Here's how the part is built. I have some questions about the finished solid (model axes, mm). A direction names the side the tool comes from. Coordinates: 2 decimals unless noted, no trailing zeros. Write each loop counter-clockwise with the first axis right and the second up, starting at its lowest first coordinate (ties: lowest second). Pieces come first, ordered by that corner, then holes. Notation, with made-up numbers: (-36, 39.25) -> (-19, 39.25) arc R21 cw to (-19, 76.25) -> close; hole circle Ø4 at (35.25, -34). An arc over 180 degrees is marked (long way). Use a Markdown table: item, result. Add a question column.
```python
from build123d import *

# Parameters (mm, degrees)
SKETCH1_W           = 7
SKETCH1_H           = 6
BOSS_EXTRUDE1_DEPTH = 9
SKETCH2_W           = 2
SKETCH2_H           = 2
SKETCH2_W_2         = 1
SKETCH2_H_2         = 3
CUT_EXTRUDE1_DEPTH  = 7
SKETCH3_OUTSIDE_W   = 11.576
SKETCH3_OUTSIDE_H   = 13.576
CUT_EXTRUDE3_DEPTH  = 3
CUT_EXTRUDE4_DEPTH  = 3
CUT_EXTRUDE5_DEPTH  = 1
SKETCH8_W           = 3
SKETCH8_H           = 3.605551275
CUT_EXTRUDE6_DEPTH  = 5.160251472


with BuildPart() as part:
    # Sketch1 → Boss-Extrude1 (new body)
    with BuildSketch(Plane.XY):
        Rectangle(SKETCH1_W, SKETCH1_H)
    extrude(amount=BOSS_EXTRUDE1_DEPTH)

    # Sketch2 → Cut-Extrude1 (cut, through all)
    with BuildSketch(Plane(origin=(0, 3, 0), x_dir=(1, 0, 0), z_dir=(0, 1, 0))):
        with Locations((-2.5, -8)):
            Rectangle(SKETCH2_W, SKETCH2_H)
        with Locations((2.5, -8)):
            Rectangle(SKETCH2_W, SKETCH2_H)
        with Locations((3, -3.5)):
            Rectangle(SKETCH2_W_2, SKETCH2_H_2)
    extrude(amount=-CUT_EXTRUDE1_DEPTH, mode=Mode.SUBTRACT)

    # Sketch3 outside → Cut-Extrude3 (cut)
    with BuildSketch(Plane(origin=(0, 3, 0), x_dir=(1, 0, 0), z_dir=(0, 1, 0))):
        with Locations((0, -4.5)):
            Rectangle(SKETCH3_OUTSIDE_W, SKETCH3_OUTSIDE_H)
        Polygon((1.5, 0), (1.5, -2), (-2.5, -2), (-2.5, -4), (-3.5, -4), (-3.5, 0), align=None, mode=Mode.SUBTRACT)
    extrude(amount=-CUT_EXTRUDE3_DEPTH, mode=Mode.SUBTRACT)

    # Sketch4 → Cut-Extrude4 (cut)
    with BuildSketch(Plane.XY.offset(2)):
        Polygon((-1.5, 3), (1.5, 0), (1.5, 3), align=None)
    extrude(amount=-CUT_EXTRUDE4_DEPTH, mode=Mode.SUBTRACT)

    # Sketch5 → Cut-Extrude5 (cut)
    with BuildSketch(Plane(origin=(3.5, 0, 0), x_dir=(0, 0, -1), z_dir=(1, 0, 0))):
        Polygon((-1, 0), (-2, -2), (-2, 0), align=None)
    extrude(amount=-CUT_EXTRUDE5_DEPTH, mode=Mode.SUBTRACT)

    # Sketch8 → Cut-Extrude6 (cut, through all)
    with BuildSketch(Plane(origin=(0, 2.769230769, 1.846153846), x_dir=(1, 0, 0), z_dir=(0, 0.832050294, 0.554700196))):
        with Locations((0, -6.795077404)):
            Rectangle(SKETCH8_W, SKETCH8_H)
    extrude(amount=CUT_EXTRUDE6_DEPTH, mode=Mode.SUBTRACT)


solid = part.part
```
Q1. Which directions (+Z, -Z, +X, -X, +Y, -Y) give clear straight access to the entire face, cutting with the end or side of a thin tool? Please do faces 1 (the flat face through (3, -1, 1.5)), 2 (the flat face through (3, -1, 5)), 3 (the flat face through (-3, 2, 4)), 4 (the flat face through (-2.5, 2, 3)).
Q2. Please list where these lines run through material, in increasing order: line 1 (Y direction, x = 0.5, z = 7); line 2 (Y direction, x = -1.5, z = 3.5); line 3 (Z direction, x = -1.25, y = 1.2).
Q3. Suppose I cut it at B-B, the plane y = -0.4. Write out the boundary of the cut face in (x, z), and give its area (3 significant figures).
Q4. Suppose I cut it at D-D, the plane x = -0.5. Write out the boundary of the cut face in (y, z).
Q5. Thinking about a two-plate mould opening in X: for faces 5 (the flat face through (3.5, -2, 6)), 6 (the flat face through (0, -1, 7.5)), 7 (the flat face through (-3, -1, 7)), 8 (the flat face through (-1.5, -2, 8)), which applies, released by +X, released by -X, zero draft, split by the parting line, or undercut?
Q6. Will these pins go through, and if not, where does the flat tip stop? pin 1 (1 mm diameter, centred on x = -2.5, y = -1, fed in from +Z); pin 2 (2.5 mm diameter, centred on x = -1, y = 2, fed in from +Z); pin 3 (2 mm diameter, centred on x = 2, y = 1.5, fed in from +Z); pin 4 (1 mm diameter, centred on y = 1.5, z = 3.5, fed in from +X).
Q7. Suppose I cut it at C-C, the plane z = 0.75. Write out the boundary of the cut face in (x, y).
Q8. Suppose I cut it at A-A, the plane x = 0.75. Write out the boundary of the cut face in (y, z).
Answer key:
| question | item | result |
|---|---|---|
| 1 | face 1 | +X, +Y |
| 1 | face 2 | +X, +Y, -Y |
| 1 | face 3 | +Z, +X, -X, +Y |
| 1 | face 4 | +Z, +X, +Y |
| 2 | line 1 | y = -3 to -0.67 |
| 2 | line 2 | y = -3 to 0 |
| 2 | line 3 | z = 0 to 2 |
| 3 | outline | (-3.5, 0) -> (3.5, 0) -> (3.5, 1.2) -> (2.5, 1.2) -> (2.5, 5) -> (3.5, 5) -> (3.5, 7) -> (1.5, 7) -> (1.5, 6.6) -> (-1.5, 6.6) -> (-1.5, 7) -> (-3.5, 7) -> close |
| 3 | area | 44.0 mm^2 |
| 4 | outline | (-3, 0) -> (2, 0) -> (2, 2) -> (0, 2) -> (0, 6) -> (-2, 9) -> (-3, 9) -> close |
| 5 | face 5 | released by +X |
| 5 | face 6 | undercut |
| 5 | face 7 | zero draft |
| 5 | face 8 | released by -X |
| 6 | pin 1 | stops at z = 7 |
| 6 | pin 2 | stops at z = 2 |
| 6 | pin 3 | passes through |
| 6 | pin 4 | stops at x = -2.5 |
| 7 | outline | (-3.5, -3) -> (3.5, -3) -> (3.5, 0) -> (1.5, 0) -> (-1.5, 3) -> (-3.5, 3) -> close |
| 8 | outline | (-3, 0) -> (0.75, 0) -> (0.75, 2) -> (0, 2) -> (0, 6) -> (-2, 9) -> (-3, 9) -> close |
